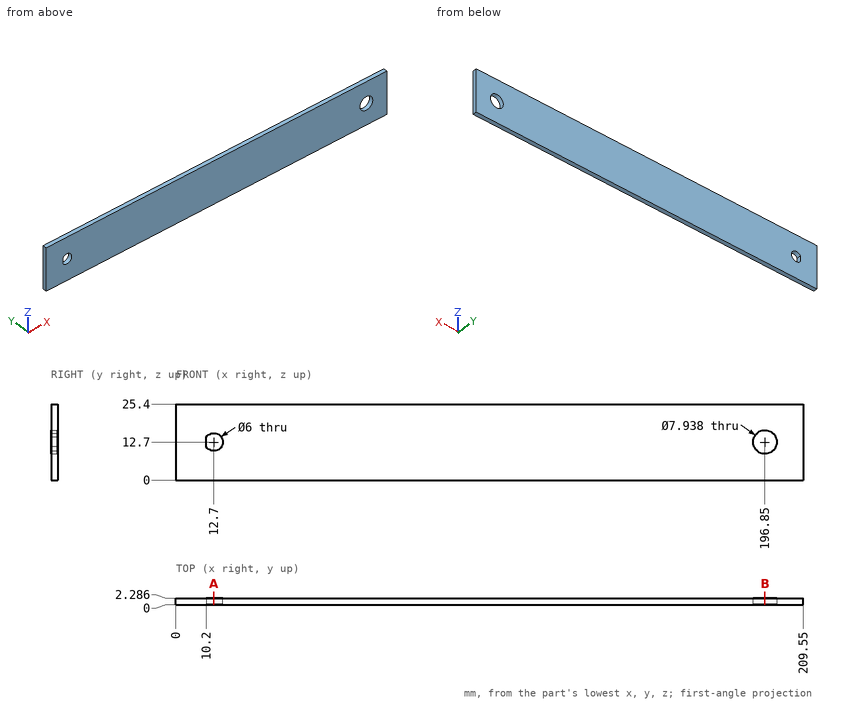
Design review of the part shown in the three views and the two pictorial views. Dimensions are in mm from the part's minimum x, y and z. Coordinates: 2 decimals unless noted, no trailing zeros. Order: outer loops, then holes, each group sorted by start corner. A loop starts at its lowest first (then second) coordinate and runs counter-clockwise, first axis right, second up. Notation, with made-up numbers: (65.25, 42) - (74.25, 42) arc R11 ccw to (74.25, 55) - close; hole circle Ø2 at (-19, -38). An arc over 180 degrees is marked (long way). Answer as CSV lines item,"result". Start each with the question number.
1) To check wall thickness, follow line 1 along X through (y, z) = (0.6, 12.7); line 2 along Z through (x, y) = (196.85, 1.1); line 3 along Z through (x, y) = (12.7, 1.8). State the ranges of each line that lie inside material, in increasing order. Write a range as [from, to].
2) Add section A-A (x = 12.7). State the section outline as (y, z) points (1 decimal).
3) Insertion check: P1, Ø1, axis at y = 1, z = 7, coming from the -X side. The pin has a flat end and moves straight along its axis. Give the tip position at first contact, or say it passes through.
4) Add section B-B (x = 196.85). State the section outline as (y, z) points (1 decimal).
Result:
1,line 1,"[0, 10.2], [15.7, 192.88], [200.82, 209.55]"
1,line 2,"[0, 8.73], [16.67, 25.4]"
1,line 3,"[0, 9.7], [15.7, 25.4]"
2,outline,"(0, 0) - (2.3, 0) - (2.3, 9.7) - (0, 9.7) - close; (0, 15.7) - (2.3, 15.7) - (2.3, 25.4) - (0, 25.4) - close"
3,P1,"x = 0"
4,outline,"(0, 0) - (2.3, 0) - (2.3, 8.7) - (0, 8.7) - close; (0, 16.7) - (2.3, 16.7) - (2.3, 25.4) - (0, 25.4) - close"
